```python
from build123d import *

# Parameters (mm, degrees)
SKETCH038_W            = 5
SKETCH038_H            = 3.1
EXTRUDE001_DEPTH       = 7
BOX010_W               = 200
BOX010_H               = 100
BOX010_DEPTH           = 100
BOX008_W               = 20
BOX008_H               = 20
BOX008_DEPTH           = 20
BOX008_PLACEMENT_ANGLE = 30
BOX011_W               = 14
BOX011_H               = 14
BOX011_DEPTH           = 20
SKETCH039_R            = 5.5
POCKET007_DEPTH        = 20.001
BOX014_W               = 7.5
BOX014_H               = 60
BOX014_DEPTH           = 200
ARRAY002_X_COUNT       = 7
ARRAY002_X_PITCH       = 47
BOX006_W               = 37
BOX006_H               = 60
BOX006_DEPTH           = 200
ARRAY_X_COUNT          = 6
ARRAY_X_PITCH          = 47
BOX012_W               = 14
BOX012_H               = 14
BOX012_DEPTH           = 12
SKETCH032_R            = 5.5
POCKET009_DEPTH        = 12.001
BOX013_W               = 14
BOX013_H               = 14
BOX013_DEPTH           = 12
SKETCH034_R            = 5.5
POCKET008_DEPTH        = 12.001
BOX009_W               = 37
BOX009_H               = 60
BOX009_DEPTH           = 200
ARRAY001_X_COUNT       = 6
ARRAY001_X_PITCH       = 47
SKETCH035_W            = 3
SKETCH035_H            = 4
SKETCH036_R            = 1.2
POCKET006_DEPTH        = 3.001


with BuildPart() as extrude001:
    # Sketch038 → Extrude001 (new body)
    with BuildSketch(Plane.YZ):
        with Locations((13.55, -28.55)):
            Rectangle(SKETCH038_W, SKETCH038_H)
    extrude(amount=EXTRUDE001_DEPTH)


with BuildPart() as bigleft:
    # Box010 → Box010 (new body)
    with BuildSketch(Plane(origin=(0, -50, -50), x_dir=(1, 0, 0), z_dir=(0, 0, 1))):
        with Locations((100, 50)):
            Rectangle(BOX010_W, BOX010_H)
    extrude(amount=BOX010_DEPTH)


with BuildPart() as pillar_cut_cube_l:
    # Box008 → Box008 (new body)
    with BuildSketch(Plane.XY):
        with Locations((10, 10)):
            Rectangle(BOX008_W, BOX008_H)
    extrude(amount=BOX008_DEPTH)


with BuildPart() as pillar_cut_cube_l_1:
    # Box008 placement: moved
    add(pillar_cut_cube_l.part.moved(Location((-127.001, 5, 20.4905))).rotate(Axis((-127.001, 5, 20.4905), (0, 1, 0)), BOX008_PLACEMENT_ANGLE))


with BuildPart() as cut011:
    # Box011 → Box011 (new body)
    with BuildSketch(Plane(origin=(-125, 8.55, 0), x_dir=(1, 0, 0), z_dir=(0, 0, 1))):
        with Locations((7, 7)):
            Rectangle(BOX011_W, BOX011_H)
    extrude(amount=BOX011_DEPTH)

    # Sketch039 → Pocket007 (cut, through all)
    with BuildSketch(Plane(origin=(-125, 8.55, 20), x_dir=(1, 0, 0), z_dir=(0, 0, 1))):
        with Locations((7, 7)):
            Circle(SKETCH039_R)
    extrude(amount=-POCKET007_DEPTH, mode=Mode.SUBTRACT)

    # Cut011: cut pillar_cut_cube_l
    add(pillar_cut_cube_l_1.part, mode=Mode.SUBTRACT)


with BuildPart() as array002:
    # Box014 → Box014 (new body)
    with BuildSketch(Plane(origin=(-128.8, 18.55, -100), x_dir=(1, 0, 0), z_dir=(0, 0, 1))):
        with Locations((3.75, 30)):
            Rectangle(BOX014_W, BOX014_H)
    extrude(amount=BOX014_DEPTH)

    # Array002 X: Array002 ×7


with BuildPart() as array002_1:
    add(array002.part)
    with Locations(*[(i * ARRAY002_X_PITCH, 0, 0) for i in range(1, ARRAY002_X_COUNT)]):
        add(array002.part)


with BuildPart() as rail_cut_cube_array_b:
    # Box006 → Box006 (new body)
    with BuildSketch(Plane(origin=(-120, 18.55, -100), x_dir=(1, 0, 0), z_dir=(0, 0, 1))):
        with Locations((18.5, 30)):
            Rectangle(BOX006_W, BOX006_H)
    extrude(amount=BOX006_DEPTH)

    # Array X: rail_cut_cube_array_b ×6


with BuildPart() as rail_cut_cube_array_b_1:
    add(rail_cut_cube_array_b.part)
    with Locations(*[(i * ARRAY_X_PITCH, 0, 0) for i in range(1, ARRAY_X_COUNT)]):
        add(rail_cut_cube_array_b.part)


with BuildPart() as cut013:
    # Sweep002: sweep along a path in Sketch028
    with BuildLine(Plane.XZ) as sweep002_path:
        Line((164.641016, 24.27441), (144.641016, 24.27441))
        ThreePointArc((144.641016, 24.27441), (123.935493, 21.548477), (104.641016, 13.556443))
        Line((104.641016, 13.556443), (70, -6.443557))
        ThreePointArc((70, -6.443557), (0, -25.2), (-70, -6.443557))
        Line((-70, -6.443557), (-130.621778, 28.556443))
    # Sketch043 → Sweep002 (sweep)
    with BuildSketch(Plane.YZ.offset(164.641016)):
        Polygon((18.55, 17.58), (47.05, 23.28), (18.55, 23.28), align=None)
    sweep(path=sweep002_path.line)

    # Cut012: cut rail_cut_cube_array_b
    add(rail_cut_cube_array_b_1.part, mode=Mode.SUBTRACT)

    # Cut013: cut Array002
    add(array002_1.part, mode=Mode.SUBTRACT)


with BuildPart() as rail_cut_b:
    # Sweep: sweep along a path in Sketch028
    with BuildLine(Plane.XZ) as sweep_path:
        Line((164.641016, 24.27441), (144.641016, 24.27441))
        ThreePointArc((144.641016, 24.27441), (123.935493, 21.548477), (104.641016, 13.556443))
        Line((104.641016, 13.556443), (70, -6.443557))
        ThreePointArc((70, -6.443557), (0, -25.2), (-70, -6.443557))
        Line((-70, -6.443557), (-130.621778, 28.556443))
    # Sketch029 → Sweep (sweep)
    with BuildSketch(Plane.YZ):
        Polygon((-19.25, -25.2), (-19.25, -31.9), (-9.25, -31.9), (-9.25, -26.2), (19.25, -26.2), (19.25, -25.2), align=None)
    sweep(path=sweep_path.line)


with BuildPart() as rail_cut_b_1:
    # Sweep placement: moved
    add(rail_cut_b.part.moved(Location((0, 27.8, 0))))

    # Cut007: cut rail_cut_cube_array_b
    add(rail_cut_cube_array_b_1.part, mode=Mode.SUBTRACT)


with BuildPart() as pillar_hollow_r:
    # Box012 → Box012 (new body)
    with BuildSketch(Plane(origin=(143, 8.55, 7), x_dir=(1, 0, 0), z_dir=(0, 0, 1))):
        with Locations((7, 7)):
            Rectangle(BOX012_W, BOX012_H)
    extrude(amount=BOX012_DEPTH)

    # Sketch032 → Pocket009 (cut, through all)
    with BuildSketch(Plane(origin=(143, 8.55, 19), x_dir=(1, 0, 0), z_dir=(0, 0, 1))):
        with Locations((7, 7)):
            Circle(SKETCH032_R)
    extrude(amount=-POCKET009_DEPTH, mode=Mode.SUBTRACT)


with BuildPart() as pillar_hollow_m:
    # Box013 → Box013 (new body)
    with BuildSketch(Plane(origin=(18, 8.55, -40), x_dir=(1, 0, 0), z_dir=(0, 0, 1))):
        with Locations((7, 7)):
            Rectangle(BOX013_W, BOX013_H)
    extrude(amount=BOX013_DEPTH)

    # Sketch034 → Pocket008 (cut, through all)
    with BuildSketch(Plane(origin=(18, 8.55, -28), x_dir=(1, 0, 0), z_dir=(0, 0, 1))):
        with Locations((7, 7)):
            Circle(SKETCH034_R)
    extrude(amount=-POCKET008_DEPTH, mode=Mode.SUBTRACT)


with BuildPart() as mount_cube_array_b:
    # Box009 → Box009 (new body)
    with BuildSketch(Plane(origin=(-120, 18.55, -100), x_dir=(1, 0, 0), z_dir=(0, 0, 1))):
        with Locations((18.5, 30)):
            Rectangle(BOX009_W, BOX009_H)
    extrude(amount=BOX009_DEPTH)

    # Array001 X: mount_cube_array_b ×6


with BuildPart() as mount_cube_array_b_1:
    add(mount_cube_array_b.part)
    with Locations(*[(i * ARRAY001_X_PITCH, 0, 0) for i in range(1, ARRAY001_X_COUNT)]):
        add(mount_cube_array_b.part)


with BuildPart() as mount_cube_array_b_2:
    # Array001 placement: moved
    add(mount_cube_array_b_1.part.moved(Location((0, -30, 0))))


with BuildPart() as clone_of_cut015:
    # Sweep001: sweep along a path in Sketch028
    with BuildLine(Plane.XZ) as sweep001_path:
        Line((-130.621778, 28.556443), (-70, -6.443557))
        ThreePointArc((-70, -6.443557), (0, -25.2), (70, -6.443557))
        Line((70, -6.443557), (104.641016, 13.556443))
        ThreePointArc((104.641016, 13.556443), (123.935493, 21.548477), (144.641016, 24.27441))
        Line((144.641016, 24.27441), (164.641016, 24.27441))
    # Sketch035 → Sweep001 (sweep)
    with BuildSketch(Plane.YZ):
        with Locations((-17.75, -33.9)):
            Rectangle(SKETCH035_W, SKETCH035_H)
    sweep(path=sweep001_path.line)


with BuildPart() as clone_of_cut015_1:
    # Sweep001 placement: moved
    add(clone_of_cut015.part.moved(Location((0, 27.8, 0))))

    # Sketch036 → Pocket006 (cut, through all)
    with BuildSketch(Plane.XZ.offset(-8.55)):
        with Locations((-127.361382, 16.612761)):
            Circle(SKETCH036_R)
        with Locations((-78.25576, -11.759304)):
            Circle(SKETCH036_R)
        with Locations((-31.170284, -30.615305)):
            Circle(SKETCH036_R)
        with Locations((15.982787, -32.973976)):
            Circle(SKETCH036_R)
        with Locations((62.801571, -19.921701)):
            Circle(SKETCH036_R)
        with Locations((109.81105, 6.487408)):
            Circle(SKETCH036_R)
        with Locations((158.314011, 15.583238)):
            Circle(SKETCH036_R)
    extrude(amount=-POCKET006_DEPTH, mode=Mode.SUBTRACT)

    # Cut010: cut mount_cube_array_b
    add(mount_cube_array_b_2.part, mode=Mode.SUBTRACT)

    # Fusion003: union Cut011, Cut013, rail_cut_b, pillar_hollow_r, pillar_hollow_m
    add(cut011.part)
    add(cut013.part)
    add(rail_cut_b_1.part)
    add(pillar_hollow_r.part)
    add(pillar_hollow_m.part)

    # Common: intersect bigleft
    add(bigleft.part, mode=Mode.INTERSECT)

    # Cut015: cut Extrude001
    add(extrude001.part, mode=Mode.SUBTRACT)


with BuildPart() as rail_fr:
    # Part__Mirroring001: instance of Clone of Cut015
    add(clone_of_cut015_1.part.mirror(Plane(origin=(82.320511, 0, -4.567103), x_dir=(1, 0, 0), z_dir=(0, 1, 0))))


with BuildPart() as rail_fr_1:
    # Part__Mirroring001 placement: moved
    add(rail_fr.part.moved(Location((0, -5, 0))))


solid = rail_fr_1.part
```
Geometry check sheet. Reference: the model listing, model coordinates, mm. A direction names the side the tool comes from. Coordinates: 2 decimals unless noted, no trailing zeros. Order: outer loops, then holes, each group sorted by start corner. A loop starts at its lowest first (then second) coordinate and runs counter-clockwise, first axis right, second up. Notation, with made-up numbers: (35.5, 37.25) - (62.5, 37.25) arc R21 cw to (62.5, 57.25) - close; hole circle Ø8 at (-14, 41.25). An arc over 180 degrees is marked (long way). Answer as a JSON object with one key per item and string values. Group by question number.
Item 1: Tool access check on faces 1 (the face through (161, -16.55, 16)), 2 (the face through (59.2, -34, -16)), 3 (the face through (19.7, -34, -27)), 4 (the face through (105, -34, 11)). Record the directions out of +Z, -Z, +X, -X, +Y, -Y that give a thin tool (end or side, any length) a straight path to the whole face; none if there is none.
Item 2: Sectioned sample at D-D, the plane x = 25. Record the cut outline in (y, z), and give its area (3 significant figures).
Item 3: Scan lines: probe 1 along X at (y, z) = (-20, -33); probe 2 along X at (y, z) = (-25, 9.5); probe 3 along X at (y, z) = (-21, 10). Record each from-to range of solid material in increasing order.
Item 4: Draft check along X on faces 5 (the face through (14, -16.55, -33)), 6 (the face through (112.434, -15.071, 5.635)), 7 (the face through (12.2, -34, -28)), 8 (the face through (115.38, -19.7, 18.73)). Enter one of: +X half, -X half, draft (parallel to the pull), parting line (faces both ways), or undercut.
Item 5: Sectioned sample at B-B, the plane y = -32.5. Give the number of separate pieces and of enclosed holes in the cut face, and give its area (3 significant figures).
Item 6: Sectioned sample at C-C, the plane z = -2. Record the cut outline in (x, y).
Item 7: Sectioned sample at A-A, the plane x = 150. Record the cut outline in (y, z).
Item 8: Depth check by flat-ended pin: pin 1 Ø1 at (y, z) = (-26, -2) entering from +X; pin 2 Ø1.9 at (y, z) = (-31.5, 13) entering from -X; pin 3 Ø13 at (x, z) = (150, 11) entering from -Y; pin 4 Ø3 at (x, z) = (62.8, -19.92) entering from -Y. Enter the tip coordinate at first touch or a pass-through.
Resolved:
{
 "1": {"face 1": "-Z, +X, -Y", "face 2": "-Z, -Y", "face 3": "-Y", "face 4": "+Z, -Z, -X, -Y"},
 "2": {"outline": "(-27.55, -40) - (-26.05, -40) - (-26.05, -28) - (-27.55, -28) - close; (-23.55, -29.75) - (-15.05, -29.75) - (-15.05, -40) - (-13.55, -40) - (-13.55, -22.95) - (-23.55, -22.95) - close", "area": "101 mm^2"},
 "3": {"probe 1": "18 to 19.53, 30.47 to 32", "probe 2": "105 to 106.2, 143 to 146.77, 153.23 to 157", "probe 3": "98.48 to 112.19, 143 to 144.52, 155.48 to 157"},
 "4": {"face 5": "undercut", "face 6": "+X half", "face 7": "undercut", "face 8": "-X half"},
 "5": {"separate pieces": "4", "enclosed holes": "0", "area": "96.7 mm^2"},
 "6": {"outline": "(77.7, -23.55) - (91.1, -23.55) - (91.1, -13.55) - (77.7, -13.55) - close"},
 "7": {"outline": "(-27.55, 7) - (-26.05, 7) - (-26.05, 19) - (-27.55, 19) - close; (-23.55, 17.57) - (-15.05, 17.57) - (-15.05, 7) - (-13.55, 7) - (-13.55, 24.27) - (-23.55, 24.27) - close"},
 "8": {"pin 1": "through", "pin 2": "x = 105", "pin 3": "y = -27.55", "pin 4": "y = -16.55"}
}
